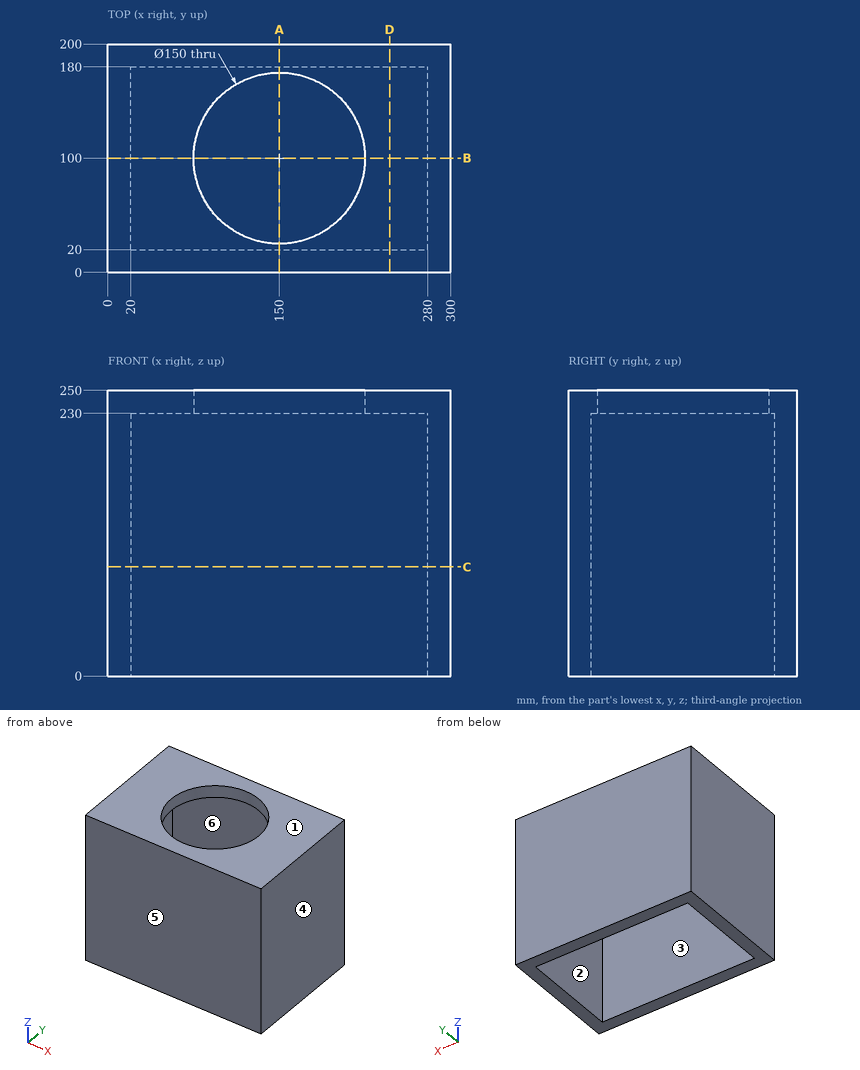
Part print with two shaded views. Sizes in mm from the minimum x, y, z corner. A direction names the side the tool comes from. Round coordinates to 2 decimals unless told otherwise and drop trailing zeros. Order: outer loops, then holes, each group sorted by start corner. A loop starts at its lowest first (then second) coordinate and runs counter-clockwise, first axis right, second up. Notation, with made-up numbers: M 26,-11 L 60,-11 A9 ccw 60,5 Z; hole C -25.5,-14 d1. An arc over 180 degrees is marked long. Answer in a Markdown table with one row per item. Add a question column.
Q1. Cut at B-B on y = 100. Give the cut face in (x, z).
Q2. Mould opens along X. For the marked faces 1, 2, 3 and 4 say: +X half, -X half, draft (parallel to the pull), parting line (faces both ways), or undercut.
Q3. Pin check, flat tips, straight feed: pin 1 (12 mm diameter, centred on x = 89, z = 36.5, fed in from -Y); pin 2 (3 mm diameter, centred on x = 67.5, y = 176.5, fed in from -Z). Stop position of each tip, or through.
Q4. Cut at C-C on z = 95.5. Give the cut face in (x, y).
Q5. 3-axis set-ups, long thin cutter, end or side, ignore diameter. For the marked faces 5 and 6: which of +Z, -Z, +X, -X, +Y, -Y reach the whole face in a straight line?
Q6. Cut at A-A on x = 150. Give the cut face in (y, z), and give its area (3 significant figures).
Q7. Wall check: L1, parallel to X at y = 105.5, z = 165.5; L2, parallel to Y at x = 180, z = 197.5; L3, parallel to Y at x = 150, z = 237. Give the ranges that are in metal, low to high. Write a range as from..to.
Q8. Cut at D-D on x = 246.5. Give the cut face in (y, z).
Established:
| question | item | result |
|---|---|---|
| 1 | outline | M 0,0 L 20,0 L 20,230 L 75,230 L 75,250 L 0,250 Z; M 225,230 L 280,230 L 280,0 L 300,0 L 300,250 L 225,250 Z |
| 2 | face 1 | draft |
| 2 | face 2 | undercut |
| 2 | face 3 | undercut |
| 2 | face 4 | +X half |
| 3 | pin 1 | stops at y = 0 |
| 3 | pin 2 | stops at z = 230 |
| 4 | outline | M 0,0 L 300,0 L 300,200 L 0,200 Z; hole M 20,20 L 280,20 L 280,180 L 20,180 Z |
| 5 | face 5 | +Z, -Z, +X, -X, -Y |
| 5 | face 6 | -Z |
| 6 | outline | M 0,0 L 20,0 L 20,230 L 25,230 L 25,250 L 0,250 Z; M 175,230 L 180,230 L 180,0 L 200,0 L 200,250 L 175,250 Z |
| 6 | area | 10,200 mm2 |
| 7 | L1 | x = 0..20, 280..300 |
| 7 | L2 | y = 0..20, 180..200 |
| 7 | L3 | y = 0..25, 175..200 |
| 8 | outline | M 0,0 L 20,0 L 20,230 L 180,230 L 180,0 L 200,0 L 200,250 L 0,250 Z |
